Here's how the part is built. I have some questions about the finished solid (model axes, mm). Give positions to 0.01 mm unless a question says otherwise; leave off trailing zeros. Loops run counter-clockwise (first coordinate to the right, second up) from the corner with the lowest first, then second, coordinate; pieces in that order, holes last. Notation, with made-up numbers: (40, 10.5) - (58, 10.5) arc R28 ccw to (58, 49.5) - close; hole circle Ø9 at (81.5, -4). An arc over 180 degrees is marked (long way). Return JSON: item names as keys, results as strings. Group by question number.
(1) For P1, Ø1, axis at x = 10, y = 6, coming from the -Z side, with a flat end and sliding along its axis, tell me the tip position at first contact or that it passes through.
(2) If we section it at B-B (y = 2): Please give me the cut outline in (x, z).
(3) If we section it at A-A (x = 15): Please give me the cut outline in (y, z), then the cut area to 3 significant figures.
(4) If we section it at C-C (y = 3.5): State how many separate pieces and enclosed holes the cut face has, then the cut area to 3 significant figures.
(5) I need wall thicknesses on probe 1 along Y at (x, z) = (2, 0.5); probe 2 along X at (y, z) = (3.25, 0.45); probe 3 along Y at (x, z) = (13.75, 0.7). Which ranges of each line are inside material? Lowest first, please. Write a range as [from, to].
```python
from build123d import *

# Parameters (mm, degrees)
ESQUISSE1_W        = 17
ESQUISSE1_H        = 8
ESQUISSE1_R        = 1.5
BOSS_EXTRU_1_DEPTH = 1
CHANFREIN1_SIZE    = 1
CONG_1_R           = 0.2


with BuildPart() as part:
    # Esquisse1 → Boss.-Extru.1 (new body)
    with BuildSketch(Plane.XY):
        with Locations((8.5, 4)):
            Rectangle(ESQUISSE1_W, ESQUISSE1_H)
        with Locations((2, 4)):
            Circle(ESQUISSE1_R, mode=Mode.SUBTRACT)
        with Locations((15, 4)):
            Circle(ESQUISSE1_R, mode=Mode.SUBTRACT)
    extrude(amount=BOSS_EXTRU_1_DEPTH)

    # Chanfrein1
    # the kernel refuses this chamfer: 1 mm, written as the material it takes off along each edge
    with BuildSketch(Plane(origin=(17, -2.571682988, 1), x_dir=(0.02749587661058563, 0, -0.9996219169112968), z_dir=(0, 1, 0)), Plane(origin=(0, 10.571682988, 1), x_dir=(-0.027495876610586372, 0, -0.9996219169112968), z_dir=(0, -1, 0))) as chanfrein1_piece_1:
        Polygon((CHANFREIN1_SIZE * 0.999621916911, CHANFREIN1_SIZE * 0.0274958766106), (-CHANFREIN1_SIZE * 0.0274958766106, CHANFREIN1_SIZE * 0.999621916911), (0, 0), align=None)
    extrude(amount=13.143365976, mode=Mode.SUBTRACT)

    # Congé1
    # the kernel refuses this fillet: 0.2 mm, written as the material it takes off along each edge
    with BuildSketch(Plane(origin=(15, 4, 0), x_dir=(1, 0, 0), z_dir=(0, -1, 0))) as cong_1_piece_1:
        with BuildLine():
            CenterArc((1.5 + CONG_1_R, CONG_1_R), CONG_1_R, 180, 90)
            Line((1.5, CONG_1_R), (1.5, 0))
            Line((1.5, 0), (1.5 + CONG_1_R, 0))
        make_face()
    revolve(axis=Axis((15, 4, 0), (0, 0, 1)), mode=Mode.SUBTRACT)
    with BuildSketch(Plane(origin=(-0.5, 0, 0), x_dir=(0, 0, 1), z_dir=(1, 0, 0))) as cong_1_piece_2:
        with BuildLine():
            CenterArc((CONG_1_R, -CONG_1_R), CONG_1_R, 90, 90)
            Line((0, -CONG_1_R), (0, 0))
            Line((0, 0), (CONG_1_R, 0))
        make_face()
    extrude(amount=18, mode=Mode.SUBTRACT)
    with BuildSketch(Plane(origin=(17, -1.207106781, 0), x_dir=(-1, 0, 0), z_dir=(0, 1, 0)), Plane(origin=(0, 9.207106781, 0), x_dir=(1, 0, 0), z_dir=(0, -1, 0))) as cong_1_piece_3:
        with BuildLine():
            CenterArc((CONG_1_R * 2.41421356237, CONG_1_R), CONG_1_R, 135, 135)
            Line((CONG_1_R * 1.70710678119, CONG_1_R * 1.70710678119), (0, 0))
            Line((0, 0), (CONG_1_R * 2.41421356237, 0))
        make_face()
    extrude(amount=10.414213562, mode=Mode.SUBTRACT)
    with BuildSketch(Plane(origin=(17.5, 8, 0), x_dir=(0, -1, 0), z_dir=(-1, 0, 0))) as cong_1_piece_4:
        with BuildLine():
            CenterArc((CONG_1_R, CONG_1_R), CONG_1_R, 180, 90)
            Line((0, CONG_1_R), (0, 0))
            Line((0, 0), (CONG_1_R, 0))
        make_face()
    extrude(amount=18, mode=Mode.SUBTRACT)
    with BuildSketch(Plane(origin=(2, 4, 0), x_dir=(1, 0, 0), z_dir=(0, -1, 0))) as cong_1_piece_5:
        with BuildLine():
            CenterArc((1.5 + CONG_1_R, CONG_1_R), CONG_1_R, 180, 90)
            Line((1.5, CONG_1_R), (1.5, 0))
            Line((1.5, 0), (1.5 + CONG_1_R, 0))
        make_face()
    revolve(axis=Axis((2, 4, 0), (0, 0, 1)), mode=Mode.SUBTRACT)
    with BuildSketch(Plane(origin=(1, 3.089072792, 1), x_dir=(1, 0, 0), z_dir=(0, -1, 0)), Plane(origin=(1, 8.207106781, 1), x_dir=(1, 0, 0), z_dir=(0, -1, 0))) as cong_1_piece_6:
        with BuildLine():
            CenterArc((CONG_1_R * 0.414213562373, -CONG_1_R), CONG_1_R, 90, 45)
            Line((-CONG_1_R * 0.292893218813, -CONG_1_R * 0.292893218813), (0, 0))
            Line((0, 0), (CONG_1_R * 0.414213562373, 0))
        make_face()
    extrude(amount=3.296179574, mode=Mode.SUBTRACT)
    with BuildSketch(Plane(origin=(2, 4, 1), x_dir=(-0.8739874769428458, -0.4859484439187749, 0), z_dir=(-0.4859484439187749, 0.8739874769428458, 0))) as cong_1_piece_7:
        with BuildLine():
            CenterArc((1.5 + CONG_1_R, -CONG_1_R), CONG_1_R, 90, 90)
            Line((1.5, -CONG_1_R), (1.5, 0))
            Line((1.5, 0), (1.5 + CONG_1_R, 0))
        make_face()
    revolve(axis=Axis((2, 4, 1), (0, 0, 1)), revolution_arc=150.925369424, mode=Mode.SUBTRACT)
    with BuildSketch(Plane(origin=(16.5, 8, 1), x_dir=(0, -1, 0), z_dir=(-1, 0, 0))) as cong_1_piece_8:
        with BuildLine():
            CenterArc((CONG_1_R, -CONG_1_R), CONG_1_R, 90, 90)
            Line((0, -CONG_1_R), (0, 0))
            Line((0, 0), (CONG_1_R, 0))
        make_face()
    extrude(amount=16, mode=Mode.SUBTRACT)
    with BuildSketch(Plane(origin=(16, 4.910927208, 1), x_dir=(0.707106781186839, 0, -0.707106781186256), z_dir=(0, 1, 0)), Plane(origin=(16, -0.207106781, 1), x_dir=(0.707106781186839, 0, -0.707106781186256), z_dir=(0, 1, 0))) as cong_1_piece_9:
        with BuildLine():
            CenterArc((CONG_1_R * 0.414213562373, CONG_1_R), CONG_1_R, 225, 45)
            Line((-CONG_1_R * 0.292893218813, CONG_1_R * 0.292893218813), (0, 0))
            Line((0, 0), (CONG_1_R * 0.414213562373, 0))
        make_face()
    extrude(amount=3.296179574, mode=Mode.SUBTRACT)
    with BuildSketch(Plane(origin=(15, 4, 1), x_dir=(0.8744070091205912, 0.48519313927629093, 0), z_dir=(0.48519313927629093, -0.8744070091205912, 0))) as cong_1_piece_10:
        with BuildLine():
            CenterArc((1.5 + CONG_1_R, -CONG_1_R), CONG_1_R, 90, 90)
            Line((1.5, -CONG_1_R), (1.5, 0))
            Line((1.5, 0), (1.5 + CONG_1_R, 0))
        make_face()
    revolve(axis=Axis((15, 4, 1), (0, 0, 1)), revolution_arc=301.949745716, mode=Mode.SUBTRACT)
    with BuildSketch(Plane(origin=(0.5, 0, 1), x_dir=(0, 0, -1), z_dir=(1, 0, 0))) as cong_1_piece_11:
        with BuildLine():
            CenterArc((CONG_1_R, CONG_1_R), CONG_1_R, 180, 90)
            Line((0, CONG_1_R), (0, 0))
            Line((0, 0), (CONG_1_R, 0))
        make_face()
    extrude(amount=16, mode=Mode.SUBTRACT)
    with BuildSketch(Plane(origin=(2, 4, 1), x_dir=(1, 0, 0), z_dir=(0, -1, 0))) as cong_1_piece_12:
        with BuildLine():
            CenterArc((1.5 + CONG_1_R, -CONG_1_R), CONG_1_R, 90, 90)
            Line((1.5, -CONG_1_R), (1.5, 0))
            Line((1.5, 0), (1.5 + CONG_1_R, 0))
        make_face()
    revolve(axis=Axis((2, 4, 1), (0, 0, 1)), revolution_arc=150.925369424, mode=Mode.SUBTRACT)


solid = part.part
```
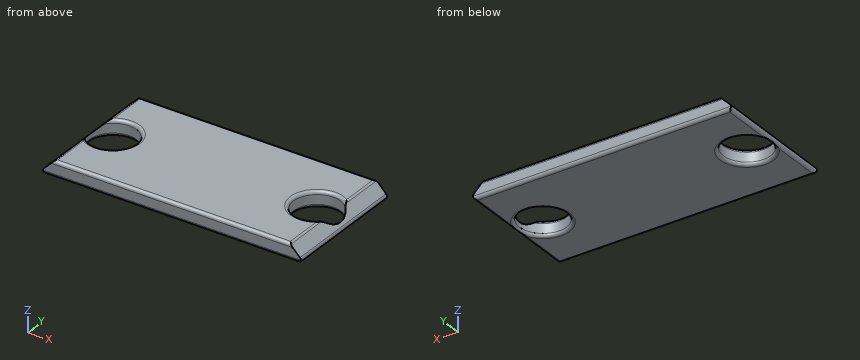
Values:
{
 "1": {"P1": "z = 0"},
 "2": {"outline": "(0.34, 0.34) arc R0.2 ccw to (0.48, 0) - (16.52, 0) arc R0.2 ccw to (16.66, 0.34) - (16.06, 0.94) arc R0.2 ccw to (15.92, 1) - (1.08, 1) arc R0.2 ccw to (0.94, 0.94) - close"},
 "3": {"outline": "(0, 0.2) arc R0.2 ccw to (0.2, 0) - (2.3, 0) arc R0.2 ccw to (2.5, 0.2) - (2.5, 0.8) arc R0.2 ccw to (2.3, 1) - (0.2, 1) arc R0.2 ccw to (0, 0.8) - close; (5.5, 0.2) arc R0.2 ccw to (5.7, 0) - (7.8, 0) arc R0.2 ccw to (8, 0.2) - (8, 0.8) arc R0.2 ccw to (7.8, 1) - (5.7, 1) arc R0.2 ccw to (5.5, 0.8) - close", "area": "4.93 mm2"},
 "4": {"separate pieces": "3", "enclosed holes": "0", "area": "10.4 mm2"},
 "5": {"probe 1": "[0, 2.5], [5.5, 8]", "probe 2": "[0.45, 0.7], [3.3, 13.7], [16.3, 16.55]", "probe 3": "[0, 3.17], [4.83, 8]"}
}
